Design review of the part built by this model. Coordinates are the model's own, in mm. A direction names the side the tool comes from. Coordinates: 2 decimals unless noted, no trailing zeros. Loops run counter-clockwise (first coordinate to the right, second up) from the corner with the lowest first, then second, coordinate; pieces in that order, holes last. Notation, with made-up numbers: (77.25, -25) - (130.25, -25) arc R26 ccw to (130.25, -4) - close; hole circle Ø3 at (70.5, 43). An arc over 180 degrees is marked (long way). Use one line per item in the form item = value. Start each with the question number.
(1) Tool access review of faces 1 (the face through (-4, 4, 230)), 2 (the face through (4, 4, 230)), 3 (the face through (-4, -4, 230)), 4 (the face through (-1.08, -4.88, 113.39)): name each direction out of +Z, -Z, +X, -X, +Y, -Y from which nothing blocks a thin tool from reaching the whole face with its end or side.
(2) Add section B-B (y = 3.25). State the section outline as (x, z) points.
(3) For L1, parallel to X at y = -0.25, z = 43.5; L2, parallel to Y at x = 3.75, z = 80, list the stretches that pass through material, from the lowest coordinate up.
(4) Add section C-C (z = 69). State the section outline as (x, y) points.
(5) Add section A-A (x = 3). State the section outline as (y, z) points.
(6) Clearance check with flat-ended pins moving along their axes: pin 1 Ø1.5 at (y, z) = (1, 71) entering from +X; pin 2 Ø5 at (y, z) = (3, 37) entering from -X. State where each tip first meets the part, or that it passes through.
```python
from build123d import *

# Parameters (mm, degrees)
F0_R     = 5
F1_DEPTH = 230
F3_DEPTH = 15


with BuildPart() as f1:
    # F0 (on Top) → F1 (new body)
    with BuildSketch(Plane.XY):
        Circle(F0_R)
    extrude(amount=F1_DEPTH)

    # F2 (on face) → F3 (join)
    with BuildSketch(Plane.XY.offset(230)):
        with BuildLine():
            ThreePointArc((-5, 0), (-3.535534, 3.535534), (0, 5))
            Line((0, 5), (-5, 5))
            Line((-5, 5), (-5, 0))
        make_face()
        with BuildLine():
            Line((5, 0), (5, 5))
            Line((5, 5), (0, 5))
            ThreePointArc((0, 5), (3.535534, 3.535534), (5, 0))
        make_face()
        with BuildLine():
            ThreePointArc((5, 0), (3.535534, 3.535534), (0, 5))
            ThreePointArc((0, 5), (-3.535534, 3.535534), (-5, 0))
            ThreePointArc((-5, 0), (-3.535534, -3.535534), (0, -5))
            ThreePointArc((0, -5), (3.535534, -3.535534), (5, 0))
        make_face()
        with BuildLine():
            Line((5, -5), (5, 0))
            ThreePointArc((5, 0), (3.535534, -3.535534), (0, -5))
            Line((0, -5), (5, -5))
        make_face()
        with BuildLine():
            ThreePointArc((0, -5), (-3.535534, -3.535534), (-5, 0))
            Line((-5, 0), (-5, -5))
            Line((-5, -5), (0, -5))
        make_face()
    extrude(amount=F3_DEPTH)


solid = f1.part
```
Computed values:
q1.face_1 = -Z, -X, +Y
q1.face_2 = -Z, +X, +Y
q1.face_3 = -Z, -X, -Y
q1.face_4 = -Z
q2.outline = (-5, 230) - (-3.8, 230) - (-3.8, 0) - (3.8, 0) - (3.8, 230) - (5, 230) - (5, 245) - (-5, 245) - close
q3.L1 = -4.99 to 4.99
q3.L2 = -3.31 to 3.31
q4.outline = circle Ø10 at (0, 0)
q5.outline = (-5, 230) - (-4, 230) - (-4, 0) - (4, 0) - (4, 230) - (5, 230) - (5, 245) - (-5, 245) - close
q6.pin_1 = 4.99
q6.pin_2 = -4.97
